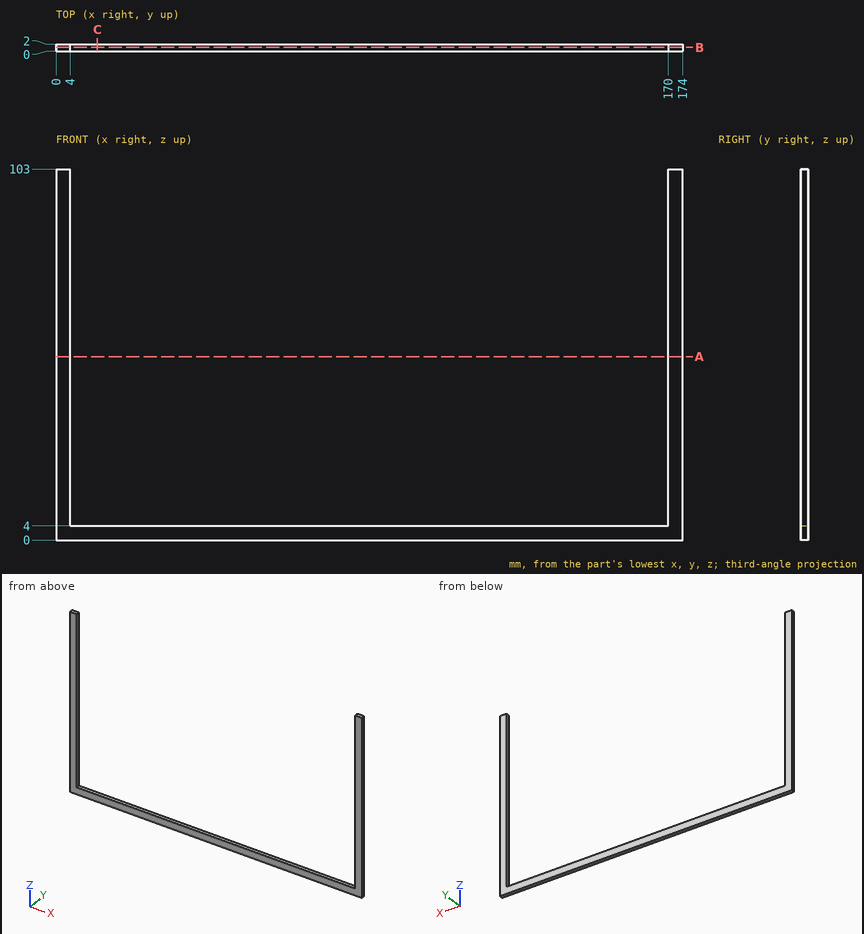
Geometry: see drawing. Coordinates: mm, zero at the bounding-box minimum. Give positions to 0.01 mm unless a question says otherwise; leave off trailing zeros. Loops run counter-clockwise (first coordinate to the right, second up) from the corner with the lowest first, then second, coordinate; pieces in that order, holes last. Notation, with made-up numbers: (-6.75, 61.5) - (4.25, 61.5) arc R8 ccw to (4.25, 65.5) - close; hole circle Ø6 at (-5, 58.5). An arc over 180 degrees is marked (long way). Use CSV: the item, a comma, the result in double quotes. Start each with the question number.
1. Section B-B (y = 1.05). Output: boundary loops of the cut face in (x, z), then the cut area to 3 significant figures.
2. Section C-C (x = 11.5). Output: boundary loops of the cut face in (y, z), then the cut area to 3 significant figures.
3. Section A-A (z = 51). Output: boundary loops of the cut face in (x, y), then the cut area to 3 significant figures.
4. Ray query, L1, parallel to X at y = 0.7, z = 9; L2, parallel to Z at x = 89, y = 1.4. Return the intervals inside material, ascending.
5. Pin query (flat end, axial travel): pin 1 (0.6 mm diameter, centred on x = 61.5, y = 1, fed in from +Z). Return the tip coordinate at first contact, or that it passes through.
Response:
1,outline,"(0, 0) - (174, 0) - (174, 103) - (170, 103) - (170, 4) - (4, 4) - (4, 103) - (0, 103) - close"
1,area,"1,490 mm²"
2,outline,"(0, 0) - (2, 0) - (2, 4) - (0, 4) - close"
2,area,"8.00 mm²"
3,outline,"(0, 0) - (4, 0) - (4, 2) - (0, 2) - close; (170, 0) - (174, 0) - (174, 2) - (170, 2) - close"
3,area,"16.0 mm²"
4,L1,"0 to 4, 170 to 174"
4,L2,"0 to 4"
5,pin 1,"z = 4"
